```python
from build123d import *

# Parameters (mm, degrees)
SKETCH_1_W      = 96
SKETCH_1_H      = 60
SKETCH_1_R      = 2.1
SKETCH_1_W_2    = 3
SKETCH_1_H_2    = 20
EXTRUDE_1_DEPTH = 6


with BuildPart() as part:
    # 草图1 → 凸台-拉伸1 (new body)
    with BuildSketch(Plane(origin=(0, 0, 0), x_dir=(1, 0, 0), z_dir=(0, 1, 0))):
        with Locations((53.5, -30)):
            Rectangle(SKETCH_1_W, SKETCH_1_H)
        with BuildLine():
            Line((72.5, -57), (34.5, -57))
            ThreePointArc((34.5, -57), (33, -55.5), (34.5, -54))
            Line((34.5, -54), (72.5, -54))
            ThreePointArc((72.5, -54), (74, -55.5), (72.5, -57))
        make_face(mode=Mode.SUBTRACT)
        with BuildLine():
            Line((72.5, -6), (34.5, -6))
            ThreePointArc((34.5, -6), (33, -4.5), (34.5, -3))
            Line((34.5, -3), (72.5, -3))
            ThreePointArc((72.5, -3), (74, -4.5), (72.5, -6))
        make_face(mode=Mode.SUBTRACT)
        with Locations(Location((76.969497546, -38, 0), (0, 0, 270))):
            Circle(SKETCH_1_R, mode=Mode.SUBTRACT)
        with Locations((62.969497546, -30)):
            Rectangle(SKETCH_1_W_2, SKETCH_1_H_2, mode=Mode.SUBTRACT)
        with Locations((97, -42)):
            Rectangle(SKETCH_1_W_2, SKETCH_1_H_2, mode=Mode.SUBTRACT)
        with Locations(Location((76.969497546, -22, 0), (0, 0, 270))):
            Circle(SKETCH_1_R, mode=Mode.SUBTRACT)
        with Locations((90.969497546, -30)):
            Rectangle(SKETCH_1_W_2, SKETCH_1_H_2, mode=Mode.SUBTRACT)
        with Locations((97, -18)):
            Rectangle(SKETCH_1_W_2, SKETCH_1_H_2, mode=Mode.SUBTRACT)
        with Locations((10, -18)):
            Rectangle(SKETCH_1_W_2, SKETCH_1_H_2, mode=Mode.SUBTRACT)
        with Locations(Location((30.030502454, -22, 0), (0, 0, 270))):
            Circle(SKETCH_1_R, mode=Mode.SUBTRACT)
        with Locations((10, -42)):
            Rectangle(SKETCH_1_W_2, SKETCH_1_H_2, mode=Mode.SUBTRACT)
        Polygon((14.530502454, -40), (14.530502454, -20), (17.530502454, -20), (17.530502454, -30), (17.530502454, -40), align=None, mode=Mode.SUBTRACT)
        with Locations(Location((30.030502454, -38, 0), (0, 0, 270))):
            Circle(SKETCH_1_R, mode=Mode.SUBTRACT)
        Polygon((42.530502454, -40), (42.530502454, -30), (42.530502454, -20), (45.530502454, -20), (45.530502454, -40), align=None, mode=Mode.SUBTRACT)
    extrude(amount=EXTRUDE_1_DEPTH)


solid = part.part
```
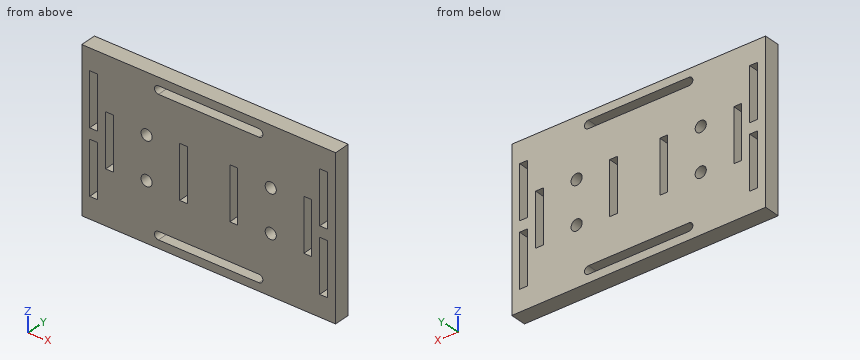
Build history of the part. All positions in model axes, mm. Coordinates: 2 decimals unless noted, no trailing zeros. Order: outer loops, then holes, each group sorted by start corner. A loop starts at its lowest first (then second) coordinate and runs counter-clockwise, first axis right, second up. Notation, with made-up numbers: M 21,12.5 L 73,12.5 A18 cw 73,33.5 Z; hole C 62,85.5 d1. An arc over 180 degrees is marked long. One line per question, with ' | ' between items. Start each with the question number.
1. Flat gauge pins, fed straight in: P1, Ø5, axis at x = 76.97, z = 38, coming from the -Y side; P2, Ø3.5, axis at x = 76.97, z = 22, coming from the -Y side. Where does each tip first touch, or does it go through?
2. Cut at B-B (z = 55.5). Write the cut outline in (x, y), plus the area to 3 significant figures.
3. Wall check: line 1 along Z through (x, y) = (46.5, 0.7); line 2 along Z through (x, y) = (10.5, 2.75); line 3 along X through (y, z) = (4.1, 40.5). Give the ranges that are in metal, low to high. Write a range as [from, to].
4. Cut at C-C (z = 17). Write the cut outline in (x, y), plus the area to 3 significant figures.
5. Cut at D-D (z = 38). Count the separate pieces of the cut face and the enclosed holes in it, plus the area to 3 significant figures.
6. Cut at A-A (x = 67). Write the cut outline in (y, z), plus the area to 3 significant figures.
The answers:
1) P1: stops at y = 0 | P2: passes through
2) outline: M 5.5,0 L 33,0 L 33,6 L 5.5,6 Z; M 74,0 L 101.5,0 L 101.5,6 L 74,6 Z | area: 330 mm2
3) line 1: z = [0, 3], [6, 54], [57, 60] | line 2: z = [0, 8], [28, 32], [52, 60] | line 3: x = [5.5, 8.5], [11.5, 95.5], [98.5, 101.5]
4) outline: M 5.5,0 L 8.5,0 L 8.5,6 L 5.5,6 Z; M 11.5,0 L 95.5,0 L 95.5,6 L 11.5,6 Z; M 98.5,0 L 101.5,0 L 101.5,6 L 98.5,6 Z | area: 540 mm2
5) separate pieces: 9 | enclosed holes: 0 | area: 418 mm2
6) outline: M 0,0 L 6,0 L 6,3 L 0,3 Z; M 0,6 L 6,6 L 6,54 L 0,54 Z; M 0,57 L 6,57 L 6,60 L 0,60 Z | area: 324 mm2
